Geometry check sheet. Reference: drawing and pictorial views, mm from the part's lowest x, y, z. Give positions to 0.01 mm unless a question says otherwise; leave off trailing zeros. Loops run counter-clockwise (first coordinate to the right, second up) from the corner with the lowest first, then second, coordinate; pieces in that order, holes last. Notation, with made-up numbers: (53.25, 47.25) -> (83.25, 47.25) arc R9 ccw to (83.25, 53.25) -> close; hole circle Ø5 at (55.25, -37). An arc over 180 degrees is marked (long way). One line per item, written item: value. Start each with the question number.
(1) Sectioned sample at B-B, the plane z = 10. Record the cut outline in (x, y).
(2) Scan lines: line 1 along X through (y, z) = (1.3, 10.5); line 2 along Z through (x, y) = (222.5, 0.6). Record each from-to range of solid material in increasing order. Write a range as from..to.
(3) Sectioned sample at C-C, the plane y = 1.1. Record the cut outline in (x, z).
(4) Sectioned sample at A-A, the plane x = 22.5. Record the cut outline in (y, z).
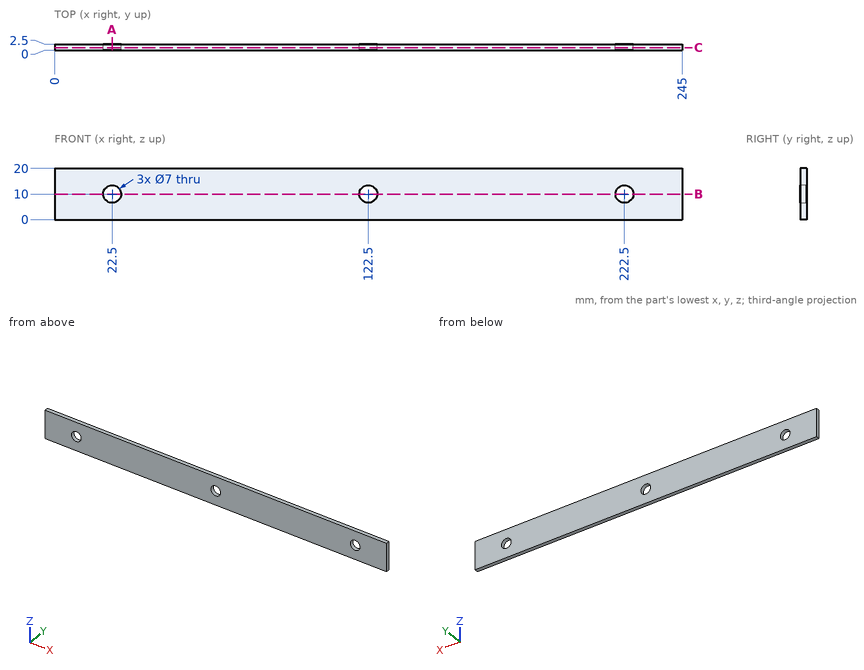
Calculated:
1. outline: (0, 0) -> (19, 0) -> (19, 2.5) -> (0, 2.5) -> close; (26, 0) -> (119, 0) -> (119, 2.5) -> (26, 2.5) -> close; (126, 0) -> (219, 0) -> (219, 2.5) -> (126, 2.5) -> close; (226, 0) -> (245, 0) -> (245, 2.5) -> (226, 2.5) -> close
2. line 1: x = 0..19.04, 25.96..119.04, 125.96..219.04, 225.96..245
2. line 2: z = 0..6.5, 13.5..20
3. outline: (0, 0) -> (245, 0) -> (245, 20) -> (0, 20) -> close; hole circle Ø7 at (22.5, 10); hole circle Ø7 at (122.5, 10); hole circle Ø7 at (222.5, 10)
4. outline: (0, 0) -> (2.5, 0) -> (2.5, 6.5) -> (0, 6.5) -> close; (0, 13.5) -> (2.5, 13.5) -> (2.5, 20) -> (0, 20) -> close
